from build123d import *

# Parameters (mm, degrees)
SKETCH1_W                                           = 17.5
SKETCH1_H                                           = 8.5
BOSS_EXTRUDE1_DEPTH                                 = 10.5
CUT_EXTRUDE1_DEPTH                                  = 21.846162716
CUT_EXTRUDE1_DEPTH_BACK                             = 21.846162716
SKETCH2_R                                           = 2.1
CHAMFER1_SIZE                                       = 0.5
CSK_FOR_M3_COUNTERSUNK_FLAT_HEAD_SCREW1_D           = 3.4
CSK_FOR_M3_COUNTERSUNK_FLAT_HEAD_SCREW1_DEPTH       = 19
CSK_FOR_M3_COUNTERSUNK_FLAT_HEAD_SCREW1_CSINK_D     = 6.3
CSK_FOR_M3_COUNTERSUNK_FLAT_HEAD_SCREW1_CSINK_ANGLE = 90
CSK_FOR_M3_COUNTERSUNK_FLAT_HEAD_SCREW1_TIP         = 1.021463052
FILLET1_R                                           = 0.5
CUT_EXTRUDE2_DEPTH                                  = 21.846162716
CUT_EXTRUDE2_DEPTH_BACK                             = 21.846162716
SKETCH6_W                                           = 21
SKETCH6_H                                           = 1
BOSS_EXTRUDE2_DEPTH                                 = 17.5
FILLET2_R                                           = 1


with BuildPart() as part:
    # Sketch1 → Boss-Extrude1 (new, symmetric)
    with BuildSketch(Plane.XY):
        Rectangle(SKETCH1_W, SKETCH1_H)
    extrude(amount=BOSS_EXTRUDE1_DEPTH, both=True)

    # Sketch2 → Cut-Extrude1 (cut, two sides: drawn at the far end of the back side and taken through both)
    with BuildSketch(Plane.ZY.offset(8.75).offset(-CUT_EXTRUDE1_DEPTH_BACK)):
        with Locations((6, -1.75)):
            Circle(SKETCH2_R)
        with Locations(Location((-6, -1.75, 0), (0, 0, 180))):
            Circle(SKETCH2_R)
        with BuildLine():
            Line((3.401923789, -3.25), (-3.401923789, -3.25))
            ThreePointArc((-3.401923789, -3.25), (-3.813859338, -3.804455891), (-4.341687605, -4.25))
            Line((-4.341687605, -4.25), (4.341687605, -4.25))
            ThreePointArc((4.341687605, -4.25), (3.813859338, -3.804455891), (3.401923789, -3.25))
        make_face()
    extrude(amount=CUT_EXTRUDE1_DEPTH + CUT_EXTRUDE1_DEPTH_BACK, mode=Mode.SUBTRACT)

    # Chamfer1
    # the kernel refuses this chamfer: 0.5 mm, written as the material it takes off along each edge
    with BuildSketch(Plane(origin=(8.75, -1.75, -6), x_dir=(0, 0, -1), z_dir=(0, 1, 0))) as chamfer1_piece_1:
        Polygon((2.1 + CHAMFER1_SIZE, 0), (2.1, CHAMFER1_SIZE), (2.1, 0), align=None)
    revolve(axis=Axis((8.75, -1.75, -6), (-1, 0, 0)), mode=Mode.SUBTRACT)
    with BuildSketch(Plane(origin=(-8.75, -1.75, -6), x_dir=(0, 0, -1), z_dir=(0, 1, 0))) as chamfer1_piece_2:
        Polygon((2.1 + CHAMFER1_SIZE, 0), (2.1, -CHAMFER1_SIZE), (2.1, 0), align=None)
    revolve(axis=Axis((-8.75, -1.75, -6), (-1, 0, 0)), mode=Mode.SUBTRACT)
    with BuildSketch(Plane(origin=(8.75, -1.75, 6), x_dir=(0, 0, 1), z_dir=(0, -1, 0))) as chamfer1_piece_3:
        Polygon((2.1 + CHAMFER1_SIZE, 0), (2.1, CHAMFER1_SIZE), (2.1, 0), align=None)
    revolve(axis=Axis((8.75, -1.75, 6), (-1, 0, 0)), mode=Mode.SUBTRACT)
    with BuildSketch(Plane(origin=(-8.75, -1.75, 6), x_dir=(0, 0, 1), z_dir=(0, -1, 0))) as chamfer1_piece_4:
        Polygon((2.1 + CHAMFER1_SIZE, 0), (2.1, -CHAMFER1_SIZE), (2.1, 0), align=None)
    revolve(axis=Axis((-8.75, -1.75, 6), (-1, 0, 0)), mode=Mode.SUBTRACT)

    # CSK for M3 Countersunk Flat Head Screw1
    with Locations(Plane(origin=(0, -3.25, 0), x_dir=(-1, 0, 0), z_dir=(0, -1, 0))):
        with Locations((4.5, 0), (-4.5, 0)):
            CounterSinkHole(CSK_FOR_M3_COUNTERSUNK_FLAT_HEAD_SCREW1_D / 2, CSK_FOR_M3_COUNTERSUNK_FLAT_HEAD_SCREW1_CSINK_D / 2, depth=CSK_FOR_M3_COUNTERSUNK_FLAT_HEAD_SCREW1_DEPTH, counter_sink_angle=CSK_FOR_M3_COUNTERSUNK_FLAT_HEAD_SCREW1_CSINK_ANGLE)
            with Locations((0, 0, -(CSK_FOR_M3_COUNTERSUNK_FLAT_HEAD_SCREW1_DEPTH + CSK_FOR_M3_COUNTERSUNK_FLAT_HEAD_SCREW1_TIP / 2))):  # 118° drill point
                Cone(0, CSK_FOR_M3_COUNTERSUNK_FLAT_HEAD_SCREW1_D / 2, CSK_FOR_M3_COUNTERSUNK_FLAT_HEAD_SCREW1_TIP, mode=Mode.SUBTRACT)

    # Fillet1
    fillet1_edges = [part.edges().sort_by_distance(p)[0] for p in [
        (2.8, 4.25, 0),
        (-6.2, 4.25, 0),
    ]]
    fillet(fillet1_edges, radius=FILLET1_R)

    # Sketch6 → Cut-Extrude2 (cut, two sides: drawn at the far end of the back side and taken through both)
    with BuildSketch(Plane.ZY.offset(8.75).offset(-CUT_EXTRUDE2_DEPTH_BACK)):
        with Locations((0, -3.75)):
            Rectangle(SKETCH6_W, SKETCH6_H)
    extrude(amount=CUT_EXTRUDE2_DEPTH + CUT_EXTRUDE2_DEPTH_BACK, mode=Mode.SUBTRACT)

    # Sketch8 → Boss-Extrude2 (add)
    with BuildSketch(Plane.ZY.offset(8.75)):
        with BuildLine():
            Line((-13.45326153, 4.25), (-10.5, 4.25))
            Line((-10.5, 4.25), (-10.5, -3.25))
            ThreePointArc((-10.5, -3.25), (-11.26491028, 0.780252897), (-13.45326153, 4.25))
        make_face()
        with BuildLine():
            Line((13.45326153, 4.25), (10.5, 4.25))
            Line((10.5, 4.25), (10.5, -3.25))
            ThreePointArc((10.5, -3.25), (11.26491028, 0.780252897), (13.45326153, 4.25))
        make_face()
    extrude(amount=-BOSS_EXTRUDE2_DEPTH)

    # Fillet2
    fillet2_edges = [part.edges().sort_by_distance(p)[0] for p in [
        (0, -3.25, 10.5),
        (0, -3.25, -10.5),
    ]]
    fillet(fillet2_edges, radius=FILLET2_R)


solid = part.part
The listing builds one solid part. Answer for the finished solid, in the listing's coordinates (mm). Coordinates: 2 decimals unless noted, no trailing zeros. Write each loop counter-clockwise with the first axis right and the second up, starting at its lowest first coordinate (ties: lowest second). Pieces come first, ordered by that corner, then holes. Notation, with made-up numbers: (26.25, -7.75) - (38.25, -7.75) arc R4 cw to (38.25, -1.75) - close; hole circle Ø8 at (43.5, 71). An arc over 180 degrees is marked (long way). Return JSON: item names as keys, results as strings.
1. For a pull along X with two mould halves and no side action, classify faces 1 (the face through (0, -3.25, 8)), 2 (the face through (-2.93, 1.01, 0.65)), 3 (the face through (8.75, 1, 0)) as +X half, -X half, draft (parallel to the pull), parting line (faces both ways), or undercut.
Final values:
{"face 1": "draft", "face 2": "undercut", "face 3": "+X half"}
2. The part is cut by section C-C on y = 3. Determine the outline of the cut face in (x, z), then the cut area to 3 significant figures.
Final values:
{"outline": "(-8.75, -12.45) - (8.75, -12.45) - (8.75, 12.45) - (-8.75, 12.45) - close; hole circle Ø3.4 at (-4.5, 0); hole circle Ø3.4 at (4.5, 0)", "area": "418 mm^2"}
3. Consider line 1 along X through (y, z) = (0.4, 0); line 2 along Z through (x, y) = (-1.5, -1.75); line 3 along X through (y, z) = (0.5, -1.25). Determine where each line is inside the solid, lowest interval first.
Final values:
{"line 1": "-8.75 to -6.2, -2.8 to 2.8, 6.2 to 8.75", "line 2": "-10.6 to -8.1, -3.9 to 3.9, 8.1 to 10.6", "line 3": "-8.75 to -5.65, -3.35 to 3.35, 5.65 to 8.75"}
4. The part is cut by section B-B on z = 0. Determine the outline of the cut face in (x, y).
Final values:
{"outline": "(-8.75, -3.25) - (-7.65, -3.25) - (-6.2, -1.8) - (-6.2, 3.75) arc R0.5 ccw to (-6.7, 4.25) - (-8.75, 4.25) - close; (-2.8, -1.8) - (-1.35, -3.25) - (1.35, -3.25) - (2.8, -1.8) - (2.8, 3.75) arc R0.5 ccw to (2.3, 4.25) - (-2.3, 4.25) arc R0.5 ccw to (-2.8, 3.75) - close; (6.2, -1.8) - (7.65, -3.25) - (8.75, -3.25) - (8.75, 4.25) - (6.7, 4.25) arc R0.5 ccw to (6.2, 3.75) - close"}
5. The part is cut by section A-A on x = 4.5. Determine the outline of the cut face in (y, z), then the cut area to 3 significant figures.
Final values:
{"outline": "(-3.25, -9.54) arc R1 ccw to (-2.33, -10.54) arc R11 cw to (4.25, -13.45) - (4.25, -2.2) arc R0.5 ccw to (3.75, -1.7) - (-1.8, -1.7) - (-3.25, -3.15) - (-3.25, -4.53) arc R2.1 cw (long way) to (-3.25, -7.47) - close; (-3.25, 3.15) - (-1.8, 1.7) - (3.75, 1.7) arc R0.5 ccw to (4.25, 2.2) - (4.25, 13.45) arc R11 cw to (-2.33, 10.54) arc R1 ccw to (-3.25, 9.54) - (-3.25, 7.47) arc R2.1 cw (long way) to (-3.25, 4.53) - close", "area": "118 mm^2"}
6. The part is cut by section D-D on z = 6. Determine the outline of the cut face in (x, y), then the cut area to 3 significant figures.
Final values:
{"outline": "(-8.75, 0.85) - (-8.25, 0.35) - (8.25, 0.35) - (8.75, 0.85) - (8.75, 4.25) - (-8.75, 4.25) - close", "area": "68.0 mm^2"}
7. Each of these flat-tipped pins is pushed along its axis until it touches: pin 1 Ø1.5 at (x, z) = (6, 5.5) entering from -Y; pin 2 Ø4.5 at (x, z) = (-4.5, 0) entering from +Y; pin 3 Ø2 at (x, y) = (-3, 2.5) entering from -Z; pin 4 Ø1.5 at (x, y) = (4.5, 2.5) entering from -Z. Where does it stop, or does it pass through?
Final values:
{"pin 1": "y = -0.06", "pin 2": "y = 4.25", "pin 3": "z = -12.81", "pin 4": "z = -12.63"}
